Read the model definition and answer for the solid it produces. Units are mm, in the model's axes. A direction names the side the tool comes from. Give positions to 0.01 mm unless a question says otherwise; leave off trailing zeros. Order: outer loops, then holes, each group sorted by start corner. A loop starts at its lowest first (then second) coordinate and runs counter-clockwise, first axis right, second up.
Item 1: A cutting plane is placed at C-C (y = 34). Write down the section's boundary in (x, z).
Item 2: A cutting plane is placed at A-A (z = 0). Write down the section's boundary in (x, y).
Item 3: A cutting plane is placed at D-D (z = 9). Write down the section's boundary in (x, y), plus the area to 3 significant figures.
Item 4: A cutting plane is placed at B-B (x = 0). Write down the section's boundary in (y, z), plus the area to 3 significant figures.
Item 5: The mould has two halves that part along Y. Classify faces 1 (the face through (7, 30, -21)), 2 (the face through (-22, 21, 2)), 3 (the face through (23, 16, -1)): +Y half, -Y half, draft (parallel to the pull), parting line (faces both ways), or undercut.
Item 6: Given pin 1 Ø4 at (x, y) = (-8.5, 35) entering from -Z; pin 2 Ø1.7 at (y, z) = (24, -21) entering from -X; pin 3 Ø1.7 at (y, z) = (27.5, 21.5) entering from +X; pin 4 Ø6 at (y, z) = (14, -1) entering from +X, each flat-ended and moving along its own axis, determine where each tip first touches the part or whether it passes through.
Item 7: Which of the six approach directions +Z, -Z, +X, -X, +Y, -Y give full straight-line access (tool end or side, diameter ignored) to faces 4 (the face through (-7, 23, 21)), 5 (the face through (22.215, 13.062, 0.189)), 6 (the face through (12.3, 55.3, 18.5))?
Item 8: Find the intervals of material crossed by line 1 along Z through (x, y) = (-0.5, -24.5); line 2 along X through (y, z) = (-26.5, 0.5); line 3 along X through (y, z) = (-6.5, -10.5), in increasing order.
Autodesk Inventor part; units mm, degrees
ref_plane "Work Plane1" through (23.5, 0, 0) normal (1, 0, 0) x (0, 1, 0)
ref_plane "XZ Plane" through (0, 0, 0) normal (0, 1, 0) x (-1, 0, 0)
ref_plane "XY Plane" through (0, 0, 0) normal (0, 0, 1) x (1, 0, 0)
sketch "Sketch1" plane through (0, 0, 0) normal (0, 0, 1) x (1, 0, 0)
  line L0 (-23.5, -60) -> (23.5, -60)
  line L1 (23.5, -60) -> (23.5, 60)
  line L2 (23.5, 60) -> (-23.5, 60)
  line L3 (-23.5, 60) -> (-23.5, -60)
  line L4 (-23.5, -60) -> (23.5, 60) construction
  line L5 (23.5, -60) -> (-23.5, 60) construction
  line L6 (-23.5, 19.5) -> (17, 60)
  line L7 (-20, -60) -> (23.5, -16.5)
  line L8 (21.5, 60) -> (21.5, -60)
  line L9 (-21.5, 60) -> (-21.5, -60)
  line L10 (0, 60) -> (0, 10.5) construction
  line L11 (-7, 60) -> (-7, 10.5)
  line L12 (7, 10.5) -> (7, 60)
  arc A0 (7, 60) -> (-7, 60) centre (0, 60) ccw
  arc A1 (-7, 10.5) -> (7, 10.5) centre (0, 10.5) ccw
  line L13 (0, 60) -> (0, -60)
  line L14 (0, -85.4) -> (0, 92.4)
  point P0 (0, 0)
  point P1 (0, 35.25)
  point P2 (-7, 36)
  point P3 (7, 50)
  dimension "d0" = 2
  dimension "d1" = 2
  dimension "d2" = 47
  dimension "d3" = 14
  dimension "d4" = 120
  dimension "d5" = 56.5
  dimension "d6" = 20
  dimension "d7" = 45
  dimension "d9" = 17
revolve "Revolution1" add sketch "Sketch1" angle 360 about axis through (0, -10, 0) along (0, 1, 0) contours L8 L7 L1 L0 | L8 L2 L1 L7
extrude "Extrusion1" cut sketch "Sketch1" along normal through all both and the other way through all contours L3 L2 L9 L6 | L7 L13 L0 | L9 L2 L11 L6 | L13 L7 L8 L0 | L11 L2 L13 L6 | L6 L13 A1 L11 | L8 L7 L1 L0 | L13 L6 L12 A1 | L13 L2 L12 L6 | A0 L14 L2 | L12 L2 L6 | L14 A0 L2
ref_plane "Work Plane1" through (23.5, 0, 0) normal (1, 0, 0) x (0, 1, 0)
sketch "Sketch2" plane through (23.5, 0, 0) normal (1, 0, 0) x (0, 1, 0)
  arc A0 (60, -16.225) -> (50, 22.4332) centre (43, 0) ccw
  line L0 (50, 22.4332) -> (10.5, 22.4332)
  line L1 (10.5, 22.4332) -> (36, 22.4332)
  arc A1 (36, 22.4332) -> (36, -22.4332) centre (43, 0) ccw
  line L2 (36, -22.4332) -> (10.5, -22.4332)
  line L3 (10.5, -22.4332) -> (50, -22.4332)
  arc A2 (50, -22.4332) -> (60, 16.225) centre (43, 0) ccw
  line L4 (60, 16.225) -> (60, -16.225)
  arc A3 (-60, -12.339) -> (-60, 12.339) centre (-40, 0) ccw
  line L5 (-60, 12.339) -> (-60, -12.339)
  line L6 (60, -16.225) -> (60, 16.225)
  line L7 (60, 0) -> (-16.5, 0)
  arc A4 (-60, -12.339) -> (-60, 12.339) centre (-40, 0) ccw
  point P0 (0, 0)
  point P1 (19.5, 0)
  point P2 (14.5, 0)
  dimension "d20" = 5
hole "Hole1" at (23.5, 14.5, 0) direction (-1, 0, 0) diameter 2.9 depth 5 counterbore diameter 5.5 counterbore depth 0.5
equation "\"d1\" = d0"
properties part number "Test_Blade_Guard"
Response values:
1. outline: (-9, -21.71) arc R23.5 ccw to (-7, -22.43) - (-7, -20.33) arc R21.5 cw to (-9, -19.53) - close; (-9, 19.53) arc R21.5 cw to (-7, 20.33) - (-7, 22.43) arc R23.5 ccw to (-9, 21.71) - close; (7, -22.43) arc R23.5 ccw to (7, 22.43) - (7, 20.33) arc R21.5 cw to (7, -20.33) - close
2. outline: (-23.5, -60) - (-21.5, -60) - (-21.5, 21.5) - (-23.5, 19.5) - close; (21.5, -18.5) - (23.5, -16.5) - (23.5, 11.75) - (23, 11.75) - (23, 13.05) - (21.5, 13.05) - close; (21.5, 15.95) - (23, 15.95) - (23, 17.25) - (23.5, 17.25) - (23.5, 60) - (21.5, 60) - close
3. outline: (-21.71, -60) - (-20, -60) - (-19.53, -59.53) - (-19.53, 23.47) - (-21.71, 21.29) - close; (19.53, -20.47) - (21.71, -18.29) - (21.71, 60) - (19.53, 60) - close
3. area: 353 mm2
4. outline: (-40, -23.5) - (3.5, -23.5) - (3.5, -21.5) - (-40, -21.5) - close; (-40, 21.5) - (3.5, 21.5) - (3.5, 23.5) - (-40, 23.5) - close
4. area: 174 mm2
5. face 1: draft
5. face 2: +Y half
5. face 3: undercut
6. pin 1: stops at z = -22.43
6. pin 2: stops at x = -12.09
6. pin 3: stops at x = 11.22
6. pin 4: stops at x = 23.5
7. face 4: +Z, -Z, +Y
7. face 5: +X
7. face 6: +Z, -Z, -X, +Y
8. line 1: z = -23.49 to -21.49, 21.49 to 23.49
8. line 2: x = -23.49 to -21.49
8. line 3: x = -21.02 to -18.76, 18.76 to 21.02
